```python
from build123d import *

# Parameters (mm, degrees)
F0_R      = 12.7
F1_DEPTH  = 20.32
F2_R      = 15.24
F5_DEPTH  = 4.191
F6_R      = 3.81
F7_DEPTH  = 63.5
F8_R      = 9.906
F9_DEPTH  = 25.4
F10_SIZE2 = 3.4892963227
F10_SIZE  = 1.27


with BuildPart() as f1:
    # F0 (on Top) → F1 (new body)
    with BuildSketch(Plane.XY):
        Circle(F0_R)
    extrude(amount=-F1_DEPTH)

    # F3 (on Front) → F4 (revolve)
    with BuildSketch(Plane.XZ):
        with BuildLine():
            Line((0, 12.7), (0, 0))
            Line((0, 0), (12.7, 0))
            ThreePointArc((12.7, 0), (8.9802561211, 8.9802561211), (0, 12.7))
        make_face()
    revolve(axis=Axis((0, 0, 6.8661598489), (0, 0, -1)))

    # F2 (on Front) → F5 (cut, symmetric)
    with BuildSketch(Plane.XZ):
        Circle(F2_R)
    extrude(amount=F5_DEPTH, both=True, mode=Mode.SUBTRACT)

    # F6 (on face) → F7 (cut, symmetric)
    with BuildSketch(Plane(origin=(0, -4.191, 0), x_dir=(-1, 0, 0), z_dir=(0, 1, 0))):
        Circle(F6_R)
    extrude(amount=F7_DEPTH, both=True, mode=Mode.SUBTRACT)

    # F8 (on face) → F9 (join)
    with BuildSketch(Plane(origin=(0, 0, -20.32), x_dir=(1, 0, 0), z_dir=(0, 0, -1))):
        Circle(F8_R)
    extrude(amount=F9_DEPTH)

    # F10
    f10_edges = [f1.edges().sort_by_distance(p)[0] for p in [
        (-9.906, 0, -45.72),
    ]]
    f10_side = f1.faces().sort_by_distance((0, 0, -45.72))[0]
    chamfer(f10_edges, length=F10_SIZE, length2=F10_SIZE2, reference=f10_side)


solid = f1.part
```
Build history of the part. All positions in model axes, mm. A direction names the side the tool comes from. Round coordinates to 2 decimals unless told otherwise and drop trailing zeros. Write each loop counter-clockwise with the first axis right and the second up, starting at its lowest first coordinate (ties: lowest second). Pieces come first, ordered by that corner, then holes.
1) Band-saw the part on D-D, the plane z = -17.5. List the corners of the cut face in (x, y).
2) Pin check, flat tips, straight feed: pin 1 (6 mm diameter, centred on x = 9.5, y = 3.5, fed in from -Z); pin 2 (2 mm diameter, centred on x = 6.5, z = 1.5, fed in from -Y); pin 3 (4 mm diameter, centred on x = 6.5, y = 10, fed in from +Z); pin 4 (2 mm diameter, centred on x = 6, y = 4.5, fed in from +Z). Stop position of each tip, or through.
3) Drill centre lines: probe 1 along Y at (x, z) = (-7.75, -11.5); probe 2 along Z at (x, y) = (0.75, -5.25); probe 3 along Y at (x, z) = (-8, 5). Where is each one in solid material? Low to high.
4) 3-axis set-ups, long thin cutter, end or side, ignore diameter. For faces 1 (the flat face through (0, -4.191, -4)), 2 (the cylindrical face through (0.83, 8.51, -3.72)): which of +Z, -Z, +X, -X, +Y, -Y reach the whole face in a straight line?
5) Band-saw the part on B-B, the plane y = 0. List the corners of the cut face in (x, z), and give its area (3 significant figures).
6) Band-saw the part on C-C, the plane z = -6. List the corners of the cut face in (x, y).
7) Band-saw the part on A-A, the plane x = 0. List the corners of the cut face in (y, z), and give its area (3 significant figures).
8) Mould opens along Y. For faces 3 (the flat face through (0, 4.191, -4)), 4 (the cylindrical face through (-1.29, -9.82, -31.12)), 5 (the flat face through (-8, -7, -20.32)) say: +Y half, -Y half, draft (parallel to the pull), parting line (faces both ways), or undercut.
Ans:
1. outline: circle Ø25.4 at (0, 0)
2. pin 1: stops at z = -45.72
2. pin 2: stops at y = -11.36
2. pin 3: stops at z = 7.92
2. pin 4: stops at z = 10.87
3. probe 1: y = -10.06 to -4.19, 4.19 to 10.06
3. probe 2: z = -45.72 to -3.74, 3.74 to 11.54
3. probe 3: y = -8.5 to -4.19, 4.19 to 8.5
4. face 1: +Z
4. face 2: +Y, -Y
5. outline: (-12.7, -20.32) - (-9.91, -20.32) - (-9.91, -42.23) - (-8.64, -45.72) - (8.64, -45.72) - (9.91, -42.23) - (9.91, -20.32) - (12.7, -20.32) - (12.7, -8.42) arc R15.24 cw to (-12.7, -8.42) - close
5. area: 679 mm2
6. outline: (-11.99, -4.19) arc R12.7 ccw to (11.99, -4.19) - close; (-11.99, 4.19) - (11.99, 4.19) arc R12.7 ccw to start
7. outline: (-12.7, -20.32) - (-9.91, -20.32) - (-9.91, -42.23) - (-8.64, -45.72) - (8.64, -45.72) - (9.91, -42.23) - (9.91, -20.32) - (12.7, -20.32) - (12.7, -3.81) - (4.19, -3.81) - (4.19, -15.24) - (-4.19, -15.24) - (-4.19, -3.81) - (-12.7, -3.81) - close; (-12.12, 3.81) - (-4.19, 3.81) - (-4.19, 11.99) arc R12.7 ccw to start; (4.19, 3.81) - (12.12, 3.81) arc R12.7 ccw to (4.19, 11.99) - close
7. area: 908 mm2
8. face 3: undercut
8. face 4: parting line
8. face 5: draft
